from build123d import *

# Parameters (mm, degrees)
F1_DEPTH = 10
F2_SIZE  = 0.5


with BuildPart() as f1:
    # F0 (on Front) → F1 (new body)
    with BuildSketch(Plane.XZ):
        Polygon((0, 1), (0, 0), (4.15, 0), (4.15, 8), (2.65, 8), (3.25, 1), align=None)
        Polygon((-4.15, 0), (0, 0), (0, 1), (-3.25, 1), (-2.65, 8), (-4.15, 8), align=None)
    extrude(amount=F1_DEPTH)

    # F2
    f2_edges = [f1.edges().sort_by_distance(p)[0] for p in [
        (-2.65, -5, 8),
        (2.65, -5, 8),
    ]]
    chamfer(f2_edges, length=F2_SIZE)


solid = f1.part
For this review, take the finished solid that the model builds, in its own axes (mm). A direction names the side the tool comes from. Give positions to 0.01 mm unless a question says otherwise; leave off trailing zeros. Order: outer loops, then holes, each group sorted by start corner. A loop starts at its lowest first (then second) coordinate and runs counter-clockwise, first axis right, second up. Notation, with made-up numbers: (8.25, 43) - (49.25, 43) arc R23 cw to (49.25, 59) - close; hole circle Ø11 at (10.5, 47.5). An arc over 180 degrees is marked (long way). Answer as a JSON object with one key per item and string values. Group by question number.
Item 1: Clearance check with a flat-ended pin moving along its axis: pin 1 Ø1 at (x, z) = (0.5, 2) entering from -Y. State where the tip first meets the part, or that it passes through.
Item 2: Take a section at B-B on y = -1.5. Give the boundary of the cut face in (x, z), and give its area (3 significant figures).
Item 3: Machinability: for faces 1 (the flat face through (0, -5, 1)), 2 (the flat face through (0, -5, 0)), which of the approach directions +Z, -Z, +X, -X, +Y, -Y give a long, thin tool a straight path to every point of the face, cutting with its end or side? Answer none if there is none.
Item 4: Draft analysis for pull direction X (two halves, no side actions). For faces 3 (the flat face through (-4, -5, 8)), 4 (the flat face through (2.967, -4.93, 4.296)), 5 (the flat face through (-4.15, -5, 4)), state which applies: pulls with the +X half, pulls with the -X half, needs draft (parallel to the pull), parting line crosses it, or undercut.
Item 5: Take a section at C-C on z = 5.25. Give the boundary of the cut face in (x, y), and give its area (3 significant figures).
Item 6: Take a section at D-D on x = 0.5. Give the boundary of the cut face in (y, z).
Item 7: Take a section at A-A on z = 2.75. Give the boundary of the cut face in (x, y).
Item 8: Wall thickness on line 1 along Z through (x, y) = (-2, -1.75); line 2 along X through (y, z) = (-7, 2); line 3 along X through (y, z) = (-4, 5.25): over which ranges is each line inside the solid? List them lowest first.
Reported:
{
 "1": {"pin 1": "through"},
 "2": {"outline": "(-4.15, 0) - (4.15, 0) - (4.15, 8) - (3.15, 8) - (2.69, 7.5) - (3.25, 1) - (-3.25, 1) - (-2.69, 7.5) - (-3.15, 8) - (-4.15, 8) - close", "area": "24.9 mm^2"},
 "3": {"face 1": "+Y, -Y", "face 2": "-Z, +X, -X, +Y, -Y"},
 "4": {"face 3": "needs draft", "face 4": "undercut", "face 5": "pulls with the -X half"},
 "5": {"outline": "(-4.15, -10) - (-2.89, -10) - (-2.89, 0) - (-4.15, 0) - close; (2.89, -10) - (4.15, -10) - (4.15, 0) - (2.89, 0) - close", "area": "25.3 mm^2"},
 "6": {"outline": "(-10, 0) - (0, 0) - (0, 1) - (-10, 1) - close"},
 "7": {"outline": "(-4.15, -10) - (-3.1, -10) - (-3.1, 0) - (-4.15, 0) - close; (3.1, -10) - (4.15, -10) - (4.15, 0) - (3.1, 0) - close"},
 "8": {"line 1": "0 to 1", "line 2": "-4.15 to -3.16, 3.16 to 4.15", "line 3": "-4.15 to -2.89, 2.89 to 4.15"}
}
